Here's how the part is built. I have some questions about the finished solid (model axes, mm). A direction names the side the tool comes from. Give positions to 0.01 mm unless a question says otherwise; leave off trailing zeros. Loops run counter-clockwise (first coordinate to the right, second up) from the corner with the lowest first, then second, coordinate; pieces in that order, holes last.
Q1. If we section it at B-B (z = 59.5): Please give me the cut outline in (x, y).
Q2. I need wall thicknesses on line 1 (Y direction, x = 0, z = 72). Which ranges of the line are inside material? Lowest first, please.
Q3. If we section it at A-A (x = 4): Please give me the cut outline in (y, z).
Q4. If we section it at D-D (x = -5.75): Please give me the cut outline in (y, z).
Q5. Will these pins go through, and if not, where does the flat tip stop? P1, Ø8, axis at x = 3, y = -37, coming from the +Z side; P2, Ø12, axis at x = 12, z = 76, coming from the +Y side; P3, Ø1, axis at x = 7.5, y = 0, coming from the +Z side.
Q6. For faces 1 (the face through (-0.1, 13.4, 100)), 2 (the face through (-1.953, 14.872, 49.3)), which set-ups out of +Z, -Z, +X, -X, +Y, -Y let a thin tool reach every point of the face, with its end or its side?
from build123d import *

# Parameters (mm, degrees)
SKETCH1_R               = 15
SKETCH1_R_2             = 13
BOSS_EXTRUDE1_DEPTH     = 100
SKETCH2_R               = 15
CUT_EXTRUDE1_DEPTH      = 100
CUT_EXTRUDE4_DEPTH      = 103.225241628
CUT_EXTRUDE4_DEPTH_BACK = 103.225241628
SKETCH3_R               = 15
SKETCH4_R               = 15
SKETCH4_R_2             = 13
BOSS_EXTRUDE3_DEPTH     = 90
BOSS_EXTRUDE4_START     = 90
SKETCH6_R               = 15
SKETCH6_R_2             = 13
BOSS_EXTRUDE4_DEPTH     = 90


with BuildPart() as part:
    # Sketch1 → Boss-Extrude1 (new body)
    with BuildSketch(Plane.XY):
        Circle(SKETCH1_R)
        Circle(SKETCH1_R_2, mode=Mode.SUBTRACT)
    extrude(amount=BOSS_EXTRUDE1_DEPTH)

    # Sketch2 → Cut-Extrude1 (cut)
    with BuildSketch(Plane(origin=(0, 0, 0), x_dir=(1, 0, 0), z_dir=(0, 1, 0))):
        Circle(SKETCH2_R)
    extrude(amount=-CUT_EXTRUDE1_DEPTH, mode=Mode.SUBTRACT)

    # Sketch3 → Cut-Extrude4 (cut, two sides: drawn at the far end of the back side and taken through both)
    with BuildSketch(Plane(origin=(0, 0, 0), x_dir=(1, 0, 0), z_dir=(0, 1, 0)).offset(-CUT_EXTRUDE4_DEPTH_BACK)):
        Circle(SKETCH3_R)
    extrude(amount=CUT_EXTRUDE4_DEPTH + CUT_EXTRUDE4_DEPTH_BACK, mode=Mode.SUBTRACT)

    # Sketch4 → Boss-Extrude3 (add)
    with BuildSketch(Plane(origin=(0, 0, 0), x_dir=(1, 0, 0), z_dir=(0, 1, 0))):
        with Locations(Location((0, 0, 0), (0, 0, 180))):
            Circle(SKETCH4_R)
        with Locations(Location((0, 0, 0), (0, 0, 90))):
            Circle(SKETCH4_R_2, mode=Mode.SUBTRACT)
    extrude(amount=BOSS_EXTRUDE3_DEPTH)

    # Sketch6 → Boss-Extrude4 (add)
    with BuildSketch(Plane.XZ.offset(BOSS_EXTRUDE4_START)):
        with Locations(Location((0, 0, 0), (0, 0, 270))):
            Circle(SKETCH6_R)
        with Locations(Location((0, 0, 0), (0, 0, 270))):
            Circle(SKETCH6_R_2, mode=Mode.SUBTRACT)
    extrude(amount=-BOSS_EXTRUDE4_DEPTH)


solid = part.part
Check sheet entries:
1. outline: circle Ø30 at (0, 0); hole circle Ø26 at (0, 0)
2. line 1: y = -15 to -13, 13 to 15
3. outline: (-90, -14.46) - (90, -14.46) - (90, -12.37) - (-90, -12.37) - close; (-90, 12.37) - (90, 12.37) - (90, 14.46) - (14.46, 14.46) - (14.46, 100) - (12.37, 100) - (12.37, 14.46) - (-12.37, 14.46) - (-12.37, 100) - (-14.46, 100) - (-14.46, 14.46) - (-90, 14.46) - close
4. outline: (-90, -13.85) - (90, -13.85) - (90, -11.66) - (-90, -11.66) - close; (-90, 11.66) - (90, 11.66) - (90, 13.85) - (13.85, 13.85) - (13.85, 100) - (11.66, 100) - (11.66, 13.85) - (-11.66, 13.85) - (-11.66, 100) - (-13.85, 100) - (-13.85, 13.85) - (-90, 13.85) - close
5. P1: stops at z = 15
5. P2: stops at y = 13.75
5. P3: stops at z = 13.27
6. face 1: +Z, +X, -X, +Y, -Y
6. face 2: +Z
